```python
from build123d import *

# Parameters (mm, degrees)
BOSS_EXTRUDE1_DEPTH = 6
SKETCH4_R           = 1.5
CUT_EXTRUDE3_DEPTH  = 4
FILLET1_R           = 5
BOSS_EXTRUDE2_DEPTH = 15


with BuildPart() as part:
    # Sketch1 → Boss-Extrude1 (new body)
    with BuildSketch(Plane(origin=(0, 0, 0), x_dir=(1, 0, 0), z_dir=(0, 1, 0))):
        Polygon((9, 21), (9, 0), (-9, 0), (-9, 21), (-5, 21), (-5, 16), (-5, 3), (5, 3), (5, 16), (5, 21), align=None)
    extrude(amount=BOSS_EXTRUDE1_DEPTH)

    # Sketch4 → Cut-Extrude3 (cut)
    with BuildSketch(Plane(origin=(0, 0, -21), x_dir=(-1, 0, 0), z_dir=(0, 0, -1))):
        with Locations((7, 3)):
            Circle(SKETCH4_R)
        with Locations(Location((-7, 3, 0), (0, 0, 180))):
            Circle(SKETCH4_R)
    extrude(amount=-CUT_EXTRUDE3_DEPTH, mode=Mode.SUBTRACT)

    # Fillet1
    fillet1_edges = [part.edges().sort_by_distance(p)[0] for p in [
        (9, 3, 0),
        (-9, 3, 0),
    ]]
    fillet(fillet1_edges, radius=FILLET1_R)

    # Sketch5 → Boss-Extrude2 (add)
    with BuildSketch(Plane.XZ):
        Polygon((4, 0), (-4, 0), (-4.783910784, -0.061833956), (-5, -0.113226949), (-5, -3), (5, -3), (5, -0.113226949), (4.783910784, -0.061833956), align=None)
    extrude(amount=-BOSS_EXTRUDE2_DEPTH)


solid = part.part
```
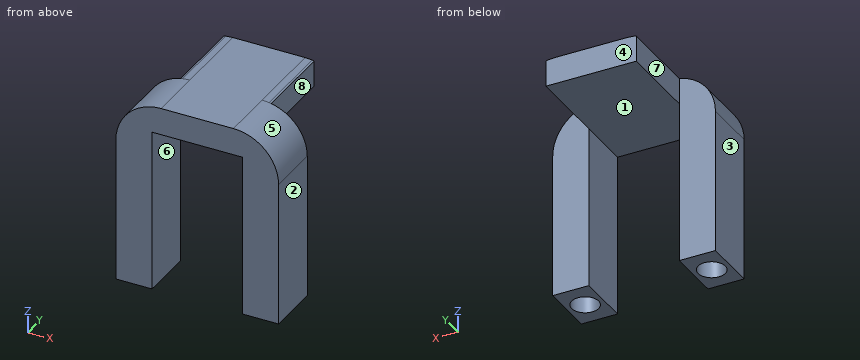
Could you check a few things on this model? Use its own coordinates, in mm. Face numbers are marked on the shaded views. A direction names the side the tool comes from. Round coordinates to 2 decimals unless told otherwise and drop trailing zeros. Loops run counter-clockwise (first coordinate to the right, second up) from the corner with the lowest first, then second, coordinate; pieces in that order, holes last.
Q1. On a 3-axis mill with a long thin cutter (end or side, diameter ignored), from which of +Z, -Z, +X, -X, +Y, -Y can I reach the whole of each face in a straight line? I mean the marked faces 4, 5, 6, 7 and 8. Say none if no direction works.
Q2. Thinking about a two-plate mould opening in X: for the marked faces 1, 2 and 3, which applies, pulls with the +X half, pulls with the -X half, needs draft (parallel to the pull), parting line crosses it, or undercut?
Q3. I want a section at A-A (z = -17.5). Write out the boundary of the cut face in (x, y), and give its area (3 significant figures).
Q4. I want a section at D-D (x = -7). Write out the boundary of the cut face in (y, z), and give its area (3 significant figures).
Q5. Please list where these lines run through material, in increasing order: L1, parallel to Y at x = -7, z = -19.65; L2, parallel to Z at x = 1.25, y = 14; L3, parallel to X at y = 10.75, z = -2.
Q6. For P1, Ø1.5, axis at x = 4, z = -10.5, coming from the -Y side; P2, Ø2.5, axis at x = 7.5, y = 3.5, coming from the -Z side; P3, Ø2.5, axis at x = 7, y = 3, coming from the -Z side; P4, Ø2.5, axis at y = 12, z = -1, coming from the +X side, each with a flat end and sliding along its axis, tell me the tip position at first contact or that it passes through.
Q7. I want a section at B-B (z = -14.25). Write out the boundary of the cut face in (x, y), and give its area (3 significant figures).
Q8. I want a section at C-C (y = 13.5). Write out the boundary of the cut face in (x, z), and give its area (3 significant figures).
Answer below:
1. face 4: +Z, -Z, +X, -X, +Y
1. face 5: +Z, +X, +Y, -Y
1. face 6: -Z, +Y, -Y
1. face 7: +Z, -Z, -X, +Y
1. face 8: +Z, -Z, +X, +Y
2. face 1: undercut
2. face 2: pulls with the +X half
2. face 3: pulls with the -X half
3. outline: (-9, 0) - (-5, 0) - (-5, 6) - (-9, 6) - close; (5, 0) - (9, 0) - (9, 6) - (5, 6) - close; hole circle Ø3 at (-7, 3); hole circle Ø3 at (7, 3)
3. area: 33.9 mm2
4. outline: (0, -21) - (1.5, -21) - (1.5, -17) - (4.5, -17) - (4.5, -21) - (6, -21) - (6, -1) - (0, -1) - close
4. area: 108 mm2
5. L1: y = 0 to 1.5, 4.5 to 6
5. L2: z = -3 to 0
5. L3: x = -5 to 5
6. P1: passes through
6. P2: stops at z = -21
6. P3: stops at z = -17
6. P4: stops at x = 5
7. outline: (-9, 0) - (-5, 0) - (-5, 6) - (-9, 6) - close; (5, 0) - (9, 0) - (9, 6) - (5, 6) - close
7. area: 48.0 mm2
8. outline: (-5, -3) - (5, -3) - (5, -0.11) - (4.78, -0.06) - (4, 0) - (-4, 0) - (-4.78, -0.06) - (-5, -0.11) - close
8. area: 29.9 mm2
